Here's how the part is built. I have some questions about the finished solid (model axes, mm). A direction names the side the tool comes from. Coordinates: 2 decimals unless noted, no trailing zeros. Write each loop counter-clockwise with the first axis right and the second up, starting at its lowest first coordinate (ties: lowest second). Pieces come first, ordered by that corner, then holes. Notation, with made-up numbers: (81.25, 62) -> (124.25, 62) arc R21 cw to (124.25, 88) -> close; hole circle Ø1 at (46, 11.5). An arc over 180 degrees is marked (long way). Put each result on its own line as item: value.
```python
from build123d import *

# Parameters (mm, degrees)
CUT_EXTRUDE3_DEPTH           = 60
CUT_EXTRUDE5_DEPTH           = 2
CUT_EXTRUDE5_DEPTH_BACK      = 30
SKETCH9_R                    = 38
SKETCH9_R_2                  = 23
SKETCH19_W                   = 12
SKETCH19_H                   = 36.5
CUT_REVOLVE2_ANGLE           = 65
CUT_REVOLVE2_OTHER_WAY_ANGLE = 65
SKETCH21_W                   = 3.25
SKETCH21_H                   = 4
BOSS_EXTRUDE3_DEPTH          = 1.35
CIRPATTERN1_COUNT            = 5
CUT_EXTRUDE9_START           = -5
CUT_EXTRUDE9_DEPTH           = 5
SKETCH23_R                   = 10.5
CUT_EXTRUDE10_DEPTH          = 10
SKETCH24_W                   = 15
SKETCH24_H                   = 8
BOSS_EXTRUDE4_DEPTH          = 8
SKETCH26_W                   = 10
SKETCH26_H                   = 6
CUT_EXTRUDE11_DEPTH          = 10
SKETCH27_W                   = 4
SKETCH27_H                   = 5
CUT_EXTRUDE12_DEPTH          = 5
CUT_EXTRUDE14_DEPTH          = 2
CUT_EXTRUDE14_DEPTH_BACK     = 30
SKETCH29_R                   = 1
CUT_EXTRUDE15_DEPTH          = 15
FILLET1_R                    = 6
FILLET2_R                    = 8
INTERSECT1_DEPTH             = 58.427876097
SKETCH31_W                   = 6
SKETCH31_H                   = 3
BOSS_EXTRUDE7_DEPTH          = 8
SKETCH32_R                   = 1
CUT_EXTRUDE16_DEPTH          = 7.5


# Read off the part's stored shape, not the designer's step: Cut-Extrude9, Intersect1
with BuildPart() as part:
    # Sketch1 → Revolve1 (revolve)
    with BuildSketch(Plane.XY, mode=Mode.PRIVATE) as revolve1_sk:
        with BuildLine():
            Line((0, 63.427876097), (32, 63.427876097))
            ThreePointArc((32, 63.427876097), (37.656854249, 61.084730346), (40, 55.427876097))
            Line((40, 55.427876097), (40, 28.846818009))
            ThreePointArc((40, 28.846818009), (38.792081772, 24.082439968), (35.460140376, 20.469057744))
            Line((35.460140376, 20.469057744), (28.539859624, 15.958818353))
            ThreePointArc((28.539859624, 15.958818353), (25.207918228, 12.345436129), (24, 7.581058088))
            Line((24, 7.581058088), (24, 3.25))
            Line((24, 3.25), (24.35, 3))
            Line((24.35, 3), (24.35, 0))
            Line((24.35, 0), (22.5, 0))
            Line((22.5, 0), (22.5, 12.5))
            ThreePointArc((22.5, 12.5), (22.353553391, 12.853553391), (22, 13))
            Line((22, 13), (0, 13))
            Line((0, 13), (0, 63.427876097))
        make_face()
    revolve(revolve1_sk.sketch.rotate(Axis((0, 0, 0), (0, 1, 0)), 90), axis=Axis((0, 0, 0), (0, 1, 0)))

    # Sketch11 → Cut-Extrude3 (cut)
    with BuildSketch(Plane(origin=(0, 13, 0), x_dir=(-1, 0, 0), z_dir=(0, -1, 0))):
        with BuildLine():
            Line((-21, 0), (21, 0))
            ThreePointArc((21, 0), (0, 21), (-21, 0))
        make_face()
    extrude(amount=-CUT_EXTRUDE3_DEPTH, mode=Mode.SUBTRACT)

    # Sketch9 → Cut-Extrude5 (cut, two sides: drawn at the far end of the back side and taken through both)
    with BuildSketch(Plane(origin=(0, 55.427876097, 0), x_dir=(1, 0, 0), z_dir=(0, 1, 0)).offset(-CUT_EXTRUDE5_DEPTH_BACK)):
        with Locations(Location((0, 0, 0), (0, 0, 270))):
            Circle(SKETCH9_R)
        with Locations(Location((0, 0, 0), (0, 0, 270))):
            Circle(SKETCH9_R_2, mode=Mode.SUBTRACT)
    extrude(amount=CUT_EXTRUDE5_DEPTH + CUT_EXTRUDE5_DEPTH_BACK, mode=Mode.SUBTRACT)

    # Sketch19 → Cut-Revolve2 (revolve, cut)
    with BuildSketch(Plane(origin=(0, 0, 0), x_dir=(0, 0, -1), z_dir=(1, 0, 0))):
        with Locations((-41.064715832, 37.177876097)):
            Rectangle(SKETCH19_W, SKETCH19_H)
    revolve(axis=Axis((0, 0, 0), (0, 1, 0)), revolution_arc=CUT_REVOLVE2_ANGLE, mode=Mode.SUBTRACT)

    # Sketch19 → Cut-Revolve2 other way (revolve, cut)
    with BuildSketch(Plane(origin=(0, 0, 0), x_dir=(0, 0, -1), z_dir=(1, 0, 0))):
        with Locations((-41.064715832, 37.177876097)):
            Rectangle(SKETCH19_W, SKETCH19_H)
    revolve(axis=Axis((0, 0, 0), (0, -1, 0)), revolution_arc=CUT_REVOLVE2_OTHER_WAY_ANGLE, mode=Mode.SUBTRACT)

    # Sketch21 → Boss-Extrude3 (add)
    with BuildSketch(Plane(origin=(0, 0, 22.5), x_dir=(-1, 0, 0), z_dir=(0, 0, -1))):
        with Locations((0, 2)):
            Rectangle(SKETCH21_W, SKETCH21_H)
    boss_extrude3 = extrude(amount=BOSS_EXTRUDE3_DEPTH)

    # CirPattern1: Boss-Extrude3 ×5 about axis
    cirpattern1_axis = Axis((0, 0, 0), (0, 1, 0))
    for i in range(1, CIRPATTERN1_COUNT):
        add(boss_extrude3.rotate(cirpattern1_axis, i * 360 / CIRPATTERN1_COUNT))

    # Cut-Extrude9 outline → Cut-Extrude9 (cut)
    with BuildSketch(Plane(origin=(0, 63.427876097, 0), x_dir=(1, 0, 0), z_dir=(0, 1, 0)).offset(CUT_EXTRUDE9_START)):
        with BuildLine():
            ThreePointArc((40, 0), (0, 40), (-40, 0))
            Line((-40, 0), (-21, 0))
            ThreePointArc((-21, 0), (0, 21), (21, 0))
            Line((21, 0), (40, 0))
        make_face()
    extrude(amount=CUT_EXTRUDE9_DEPTH, mode=Mode.SUBTRACT)

    # Sketch23 → Cut-Extrude10 (cut)
    with BuildSketch(Plane(origin=(0, 0, -40), x_dir=(-1, 0, 0), z_dir=(0, 0, -1))):
        with Locations((0, 42.137876097)):
            Circle(SKETCH23_R)
    extrude(amount=-CUT_EXTRUDE10_DEPTH, mode=Mode.SUBTRACT)

    # Sketch24 → Boss-Extrude4 (add)
    with BuildSketch(Plane(origin=(0, 58.427876097, 0), x_dir=(1, 0, 0), z_dir=(0, 1, 0))):
        with Locations((0, 30)):
            Rectangle(SKETCH24_W, SKETCH24_H)
    extrude(amount=-BOSS_EXTRUDE4_DEPTH)

    # Sketch26 → Cut-Extrude11 (cut)
    with BuildSketch(Plane(origin=(0, 58.427876097, 0), x_dir=(1, 0, 0), z_dir=(0, 1, 0))):
        with Locations((0, 30)):
            Rectangle(SKETCH26_W, SKETCH26_H)
    extrude(amount=-CUT_EXTRUDE11_DEPTH, mode=Mode.SUBTRACT)

    # Sketch27 → Cut-Extrude12 (cut)
    with BuildSketch(Plane(origin=(7.5, 0, 0), x_dir=(0, 0, -1), z_dir=(1, 0, 0))):
        with Locations((30, 53.927876097)):
            Rectangle(SKETCH27_W, SKETCH27_H)
    extrude(amount=-CUT_EXTRUDE12_DEPTH, mode=Mode.SUBTRACT)

    # Sketch28 → Cut-Extrude14 (cut, two sides: drawn at the far end of the back side and taken through both)
    with BuildSketch(Plane(origin=(0, 55.427876097, 0), x_dir=(1, 0, 0), z_dir=(0, 1, 0)).offset(-CUT_EXTRUDE14_DEPTH_BACK)):
        with BuildLine():
            Line((-22.912878475, -2), (22.912878475, -2))
            ThreePointArc((22.912878475, -2), (0, -23), (-22.912878475, -2))
        make_face()
    extrude(amount=CUT_EXTRUDE14_DEPTH + CUT_EXTRUDE14_DEPTH_BACK, mode=Mode.SUBTRACT)

    # Sketch29 → Cut-Extrude15 (cut)
    with BuildSketch(Plane(origin=(0, 0, 0), x_dir=(-1, 0, 0), z_dir=(0, 0, -1))):
        with Locations((-30.416198487, 60.927876097)):
            Circle(SKETCH29_R)
        with Locations((30.416198487, 60.927876097)):
            Circle(SKETCH29_R)
        with Locations((0, 60.927876097)):
            Circle(SKETCH29_R)
    extrude(amount=-CUT_EXTRUDE15_DEPTH, mode=Mode.SUBTRACT)

    # Fillet1
    fillet1_edges = [part.edges().sort_by_distance(p)[0] for p in [
        (21, 35.713938048, 0),
        (-21, 35.713938048, 0),
    ]]
    fillet(fillet1_edges, radius=FILLET1_R)

    # Fillet2
    fillet2_edges = [part.edges().sort_by_distance(p)[0] for p in [
        (-22.912878475, 41.427876097, 2),
        (22.912878475, 41.427876097, 2),
    ]]
    fillet(fillet2_edges, radius=FILLET2_R)

    # Intersect1 outline → Intersect1 (cut)
    with BuildSketch(Plane(origin=(0, 0, 0), x_dir=(1, 0, 0), z_dir=(0, 1, 0))):
        with BuildLine():
            Line((-37.508702776, -13.895942431), (-42, -15.355253362))
            Line((-42, -15.355253362), (-42, -41))
            Line((-42, -41), (42, -41))
            Line((42, -41), (42, -15.355253362))
            Line((42, -15.355253362), (37.508702776, -13.895942431))
            ThreePointArc((37.508702776, -13.895942431), (0, 40), (-37.508702776, -13.895942431))
        make_face()
        with BuildLine():
            ThreePointArc((19.246817919, 8.4), (18.767687244, 2.713664655), (13.747727085, 0))
            Line((13.747727085, 0), (-13.747727085, 0))
            ThreePointArc((-13.747727085, 0), (-18.767687244, 2.713664655), (-19.246817919, 8.4))
            ThreePointArc((-19.246817919, 8.4), (0, 21), (19.246817919, 8.4))
        make_face(mode=Mode.SUBTRACT)
    extrude(amount=INTERSECT1_DEPTH, mode=Mode.SUBTRACT)

    # Sketch31 → Boss-Extrude7 (add)
    with BuildSketch(Plane(origin=(0, 58.427876097, 0), x_dir=(1, 0, 0), z_dir=(0, 1, 0))):
        with Locations((0, -30)):
            Rectangle(SKETCH31_W, SKETCH31_H)
    extrude(amount=-BOSS_EXTRUDE7_DEPTH)

    # Sketch32 → Cut-Extrude16 (cut)
    with BuildSketch(Plane(origin=(3, 0, 0), x_dir=(0, 0, -1), z_dir=(1, 0, 0))):
        with Locations((-30, 54.427876097)):
            Circle(SKETCH32_R)
    extrude(amount=-CUT_EXTRUDE16_DEPTH, mode=Mode.SUBTRACT)


solid = part.part
```
Item 1: Which directions (+Z, -Z, +X, -X, +Y, -Y) give clear straight access to the entire face, cutting with the end or side of a thin tool? Please do faces 4 (the flat face through (0, 54, 28.5)), 5 (the flat face through (0, 54, 31.5)), 6 (the cylindrical face through (0.042, 53.452, 30.217)), 7 (the flat face through (0, 61, 15)), 8 (the flat face through (-3, 55, 31)).
Output:
face 4: -Z, +X, -X, -Y
face 5: +Z, +X, -X, -Y
face 6: +X, -X
face 7: -Z
face 8: +Z, -Z, -X, -Y
Item 2: Imagine slicing it at A-A on x = 0. Write out the boundary of the cut face in (y, z).
Output:
outline: (50.43, 28.5) -> (58.43, 28.5) -> (58.43, 0) -> (59.93, 0) -> (59.93, 15) -> (61.93, 15) -> (61.93, 0) -> (63.43, 0) -> (63.43, 32) arc R8 ccw to (58.43, 39.42) -> (58.43, 31.5) -> (50.43, 31.5) -> close; hole circle Ø2 at (54.43, 30)
Item 3: Please list where these lines run through material, in increasing order: line 1 along Y through (x, z) = (1.1, 30); line 2 along Y through (x, z) = (29, 7); line 3 along Z through (x, y) = (-1, 54.5). Write a range as from..to.
Output:
line 1: y = 50.43..53.43, 55.43..63.43
line 2: y = 58.43..63.43
line 3: z = 28.5..29, 31..31.5
Item 4: For P1, Ø1.2, axis at y = 54.43, z = 30, coming from the +X side; P2, Ø5, axis at x = 0.5, y = 55, coming from the +Z side; P3, Ø2.5, axis at y = 53.5, z = 30, coming from the -X side; P4, Ø3, axis at x = -30.42, y = 60.93, coming from the -Z side, each with a flat end and sliding along its axis, tell me the tip position at first contact or that it passes through.
Output:
P1: passes through
P2: stops at z = 31.5
P3: stops at x = -3
P4: stops at z = 0
Item 5: If we mould it in two halves opening along Y, with no side actions, what happens to faces 1 (the flat face through (3, 55, 31)), 2 (the cylindrical face through (-30.2, 59.95, 7.4)), 3 (the flat face through (0, 50.428, 30))? For each: released by +Y, released by -Y, zero draft, split by the parting line, or undercut.
Output:
face 1: zero draft
face 2: undercut
face 3: released by -Y
Item 6: Imagine slicing it at B-B on z = 6.5. State how many separate pieces and enclosed holes the cut face has, then the cut area to 3 significant figures.
Output:
separate pieces: 1
enclosed holes: 3
area: 359 mm²
